```python
from build123d import *

# Parameters (mm, degrees)
F1_R      = 17.75
F1_R_2    = 5
F2_DEPTH  = 9
F3_R      = 2
F4_DEPTH  = 25
F5_R      = 4.5
F6_DEPTH  = 4
F7_R      = 4.9962350467
F8_DEPTH  = 9
F10_DEPTH = 25
F12_DEPTH = 25


with BuildPart() as f2:
    # F1 (on Top) → F2 (new body)
    with BuildSketch(Plane.XY):
        Circle(F1_R)
        with Locations((0, -9.75)):
            Circle(F1_R_2, mode=Mode.SUBTRACT)
        with BuildLine():
            ThreePointArc((0, 4.75), (-3.5355339059, 13.2855339059), (5, 9.75))
            ThreePointArc((5, 9.75), (3.5355339059, 6.2144660941), (0, 4.75))
        make_face(mode=Mode.SUBTRACT)
    extrude(amount=F2_DEPTH)

    # F3 (on face) → F4 (cut)
    with BuildSketch(Plane.XY.offset(9)):
        with BuildLine():
            ThreePointArc((9.25, 0), (11.25, -2), (13.25, 0))
            ThreePointArc((13.25, 0), (11.25, 2), (9.25, 0))
        make_face()
        with Locations((-11.25, 0)):
            Circle(F3_R)
    extrude(amount=-F4_DEPTH, mode=Mode.SUBTRACT)

    # F5 (on face) → F6 (cut)
    with BuildSketch(Plane.XY.offset(9)):
        with Locations((11.25, 0)):
            Circle(F5_R)
        with Locations((-11.25, 0)):
            Circle(F5_R)
    extrude(amount=-F6_DEPTH, mode=Mode.SUBTRACT)

    # F7 (on face) → F8 (join)
    with BuildSketch(Plane.XY.offset(9)):
        with Locations((11.25, 0)):
            Circle(F7_R)
    extrude(amount=-F8_DEPTH)

    # F9 (on face) → F10 (cut)
    with BuildSketch(Plane.XY.offset(9)):
        with BuildLine():
            ThreePointArc((8.35, 0), (9.5, -1.15), (10.65, 0))
            ThreePointArc((10.65, 0), (9.5, 1.15), (8.35, 0))
        make_face()
    extrude(amount=-F10_DEPTH, mode=Mode.SUBTRACT)

    # F11 (on face) → F12 (cut)
    with BuildSketch(Plane.XY.offset(9)):
        with BuildLine():
            Line((-7.4342581112, 17.1842581112), (0, 9.75))
            Line((0, 9.75), (3.5355339059, 6.2144660941))
            Line((3.5355339059, 6.2144660941), (3.5355339059, -6.2144660941))
            Line((3.5355339059, -6.2144660941), (0, -9.75))
            Line((0, -9.75), (-7.4342581112, -17.1842581112))
            ThreePointArc((-7.4342581112, -17.1842581112), (18.7234323909, 0), (-7.4342581112, 17.1842581112))
        make_face()
    extrude(amount=-F12_DEPTH, mode=Mode.SUBTRACT)


solid = f2.part
```
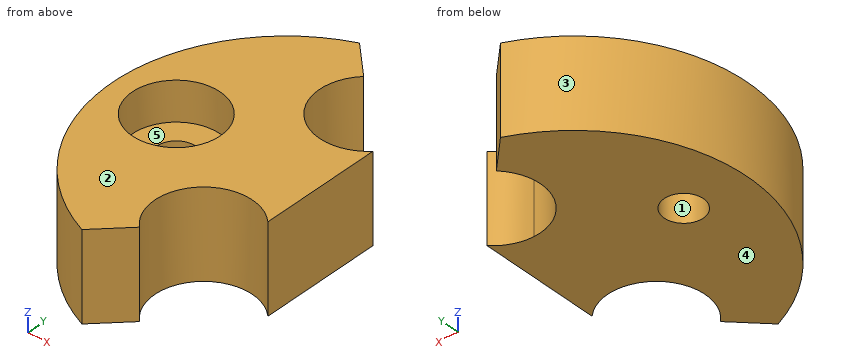
Source: CAD feature listing. Evaluate the final solid. Frame: model axes, mm. Face numbers are marked on the shaded views. A direction names the side the tool comes from. Coordinates: 2 decimals unless noted, no trailing zeros. Write each loop counter-clockwise with the first axis right and the second up, starting at its lowest first coordinate (ties: lowest second). Pieces come first, ordered by that corner, then holes. Notation, with made-up numbers: M -3.5,43.25 L 42.5,43.25 A16 cw 42.5,57.25 Z; hole C 55,57.5 d3. An arc over 180 degrees is marked long. Answer as a JSON object with one key per item and string values.
1. Cut plane C-C on x = -11.25. Output: boundary loops of the cut face in (y, z).
Evaluation:
{"outline": "M -13.73,0 L -2,0 L -2,5 L -4.5,5 L -4.5,9 L -13.73,9 Z; M 2,0 L 13.73,0 L 13.73,9 L 4.5,9 L 4.5,5 L 2,5 Z"}
2. Cut plane B-B on z = 8.25. Output: boundary loops of the cut face in (x, y).
Evaluation:
{"outline": "M -6.69,-16.44 L -3.54,-13.29 A5 cw 3.54,-6.21 L 3.54,6.21 A5 cw -3.54,13.29 L -6.69,16.44 A17.75 ccw Z; hole C -11.25,0 d9"}
3. Cut plane D-D on z = 3. Output: boundary loops of the cut face in (x, y), plus the area to 3 significant figures.
Evaluation:
{"outline": "M -6.69,-16.44 L -3.54,-13.29 A5 cw 3.54,-6.21 L 3.54,6.21 A5 cw -3.54,13.29 L -6.69,16.44 A17.75 ccw Z; hole C -11.25,0 d4", "area": "404 mm^2"}
4. Contact query for flat-ended pins moving along their axis: P1, Ø1, axis at x = -4.5, z = 3, coming from the -Y side; P2, Ø1.5, axis at y = 12.5, z = 1, coming from the -X side; P3, Ø1, axis at x = -12, z = 3.5, coming from the -Y side. Output: stop coordinate, or through.
Evaluation:
{"P1": "y = -14.75", "P2": "x = -13.3", "P3": "y = -13.52"}
5. Access query for the marked faces 4 and 5. Directions: +Z, -Z, +X, -X, +Y, -Y. A direction counts if a zero-diameter tool reaches every point of the face in a straight line with its end or side. Return the directions, or none.
Evaluation:
{"face 4": "-Z, +X, -X, +Y, -Y", "face 5": "+Z"}
6. Cut plane A-A on y = 0. Output: boundary loops of the cut face in (x, z), plus the area to 3 significant figures.
Evaluation:
{"outline": "M -17.75,0 L -13.25,0 L -13.25,5 L -15.75,5 L -15.75,9 L -17.75,9 Z; M -9.25,0 L 3.54,0 L 3.54,9 L -6.75,9 L -6.75,5 L -9.25,5 Z", "area": "136 mm^2"}
7. Draft query along Y for the marked faces 1, 2 and 3. Return one class per face: released by +Y, released by -Y, zero draft, split by the parting line, or undercut.
Evaluation:
{"face 1": "undercut", "face 2": "zero draft", "face 3": "split by the parting line"}
8. Ray query, L1, parallel to Y at x = -4, z = 7; L2, parallel to Y at x = -11.25, z = 1.75; L3, parallel to Y at x = -4.25, z = 8. Return the intervals inside material, ascending.
Evaluation:
{"L1": "-13.75 to -12.75, -6.75 to 6.75, 12.75 to 13.75", "L2": "-13.73 to -2, 2 to 13.73", "L3": "-14 to -12.38, -7.12 to 7.12, 12.38 to 14"}
